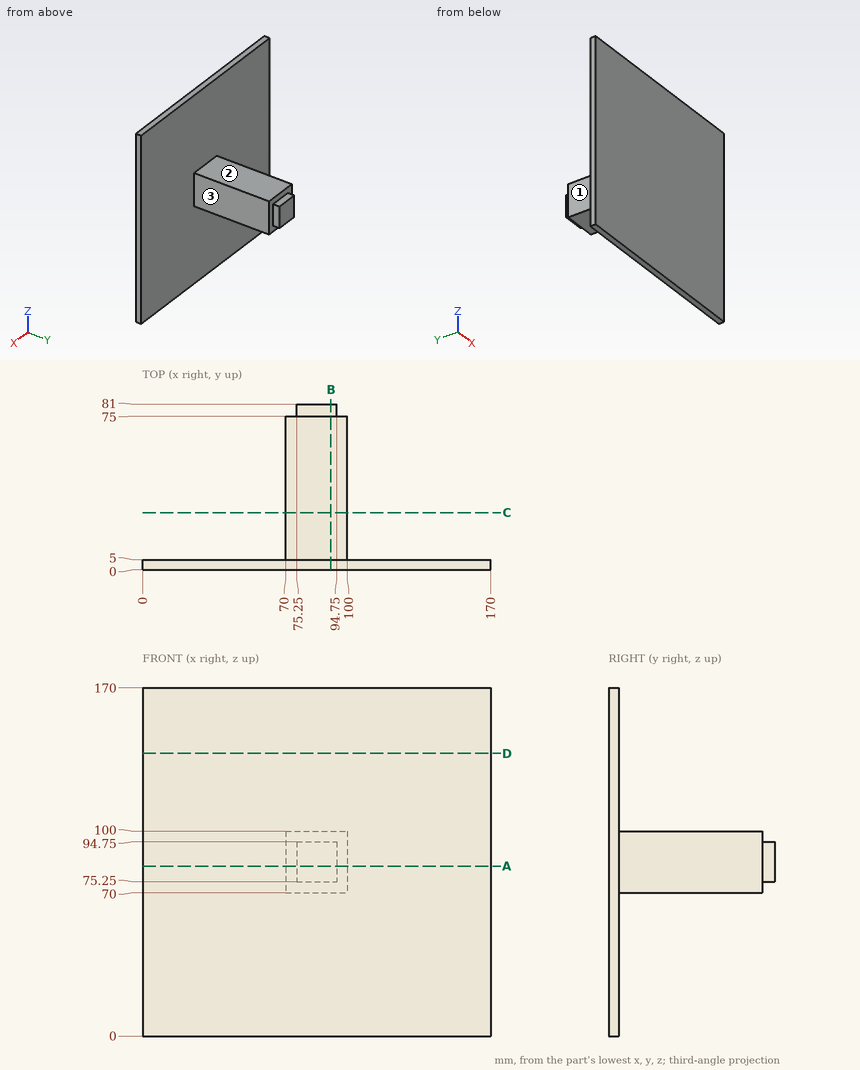
Print and shaded views of the part. All mm, measured from the part's lowest x, y and z. Coordinates: 2 decimals unless noted, no trailing zeros. Loops run counter-clockwise (first coordinate to the right, second up) from the corner with the lowest first, then second, coordinate; pieces in that order, holes last. Notation, with made-up numbers: (42.25, 88.5) - (62.25, 88.5) arc R21 ccw to (62.25, 105.5) - close; hole circle Ø1 at (-28.5, -30). An arc over 180 degrees is marked (long way). Write item = value, one per line. Start each with the question number.
Item 1: Saw through at B-B, the plane x = 92. List the corners of the cut face in (y, z), then the cut area to 3 significant figures.
Item 2: Saw through at D-D, the plane z = 138. List the corners of the cut face in (x, y), then the cut area to 3 significant figures.
Item 3: Wall check: probe 1 along Y at (x, z) = (138, 29.5); probe 2 along Z at (x, y) = (99.5, 62). Give the ranges that are in metal, low to high. Write a range as [from, to].
Item 4: Saw through at C-C, the plane y = 28. List the corners of the cut face in (x, z), then the cut area to 3 significant figures.
Item 5: Pull direction X, two halves, no side cores. Call the marked faces 1, 2 and 3: +X half, -X half, draft (parallel to the pull), parting line (faces both ways), or undercut.
Item 6: Drop flat-ended pins along their axis: pin 1 Ø4 at (x, z) = (31, 43.5) entering from +Y; pin 2 Ø6.5 at (y, z) = (79, 86) entering from -X; pin 3 Ø9 at (y, z) = (43.5, 89.5) entering from -X. Give the stop position or say it passes through.
Item 7: Saw through at A-A, the plane z = 83. List the corners of the cut face in (x, y), then the cut area to 3 significant figures.
Answers:
q1.outline = (0, 0) - (5, 0) - (5, 70) - (75, 70) - (75, 75.25) - (81, 75.25) - (81, 94.75) - (75, 94.75) - (75, 100) - (5, 100) - (5, 170) - (0, 170) - close
q1.area = 3,070 mm2
q2.outline = (0, 0) - (170, 0) - (170, 5) - (0, 5) - close
q2.area = 850 mm2
q3.probe_1 = [0, 5]
q3.probe_2 = [70, 100]
q4.outline = (70, 70) - (100, 70) - (100, 100) - (70, 100) - close
q4.area = 900 mm2
q5.face_1 = -X half
q5.face_2 = draft
q5.face_3 = +X half
q6.pin_1 = 5
q6.pin_2 = 75.25
q6.pin_3 = 70
q7.outline = (0, 0) - (170, 0) - (170, 5) - (100, 5) - (100, 75) - (94.75, 75) - (94.75, 81) - (75.25, 81) - (75.25, 75) - (70, 75) - (70, 5) - (0, 5) - close
q7.area = 3,070 mm2
